The listing builds one solid part. Answer for the finished solid, in the listing's coordinates (mm). Face numbers are marked on the shaded views. A direction names the side the tool comes from. Round coordinates to 2 decimals unless told otherwise and drop trailing zeros. Loops run counter-clockwise (first coordinate to the right, second up) from the corner with the lowest first, then second, coordinate; pieces in that order, holes last. Notation, with made-up numbers: (40, -5) -> (78, -5) arc R27 cw to (78, 26) -> close; hole circle Ø1 at (-17.5, -15). An arc over 180 degrees is marked (long way). Use a Markdown table: item, result. Add a question column.
Q1. Section B-B on z = 25 is taken. Give the vertices of the cut face in (x, y).
Q2. Section A-A on x = 29.5 is taken. Give the vertices of the cut face in (y, z), then the cut area to 3 significant figures.
Q3. Consider line 1 (X direction, y = 5, z = 33); line 2 (Y direction, x = -16, z = 7.5); line 3 (X direction, y = 17, z = 5.5). Determine where each line is inside the solid, lowest interval first.
Q4. Section D-D on z = 5.5 is taken. Give the vertices of the cut face in (x, y).
Q5. For a pull along Y with two mould halves and no side action, classify the marked faces 3, 4 and 5 as released by +Y, released by -Y, zero draft, split by the parting line, or undercut.
Q6. Section C-C on y = 22 is taken. Give the vertices of the cut face in (x, z).
Q7. Given pin 1 Ø3 at (x, y) = (33, 14) entering from +Z; pin 2 Ø4 at (x, z) = (-42, 11.5) entering from +Y; pin 3 Ø1.8 at (x, z) = (-42.5, 9.5) entering from -Y, each flat-ended and moving along its own axis, determine where each tip first touches the part or whether it passes through.
Q8. Which of the six approach directions +Z, -Z, +X, -X, +Y, -Y give full straight-line access (tool end or side, diameter ignored) to the marked faces 1 and 2?
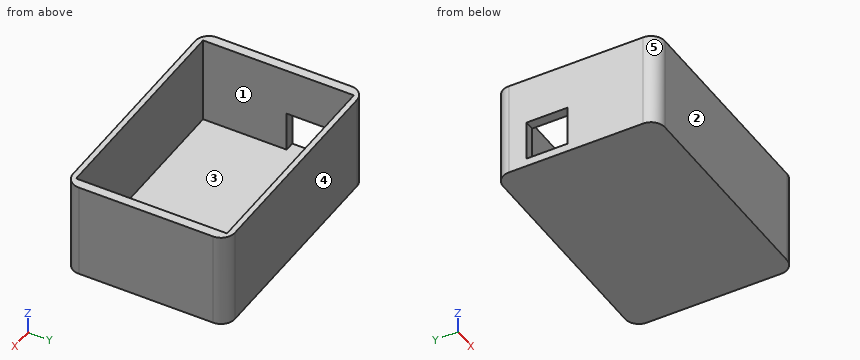
from build123d import *

# Parameters (mm, degrees)
F0_W     = 87
F0_H     = 59
F1_DEPTH = 35
F2_W     = 40
F2_H     = 27.5
F3_DEPTH = 32
F4_R     = 5
F5_W     = 15
F5_H     = 12.435101904
F5_H_2   = 2.1998170093
F6_DEPTH = 25


with BuildPart() as f1:
    # F0 (on Top) → F1 (new body)
    with BuildSketch(Plane.XY):
        Rectangle(F0_W, F0_H)
    extrude(amount=F1_DEPTH)

    # F2 (on face) → F3 (cut)
    with BuildSketch(Plane.XY.offset(35)):
        with Locations((-20, -13.75)):
            Rectangle(F2_W, F2_H)
        with Locations((20, 13.75)):
            Rectangle(F2_W, F2_H)
        with Locations((20, -13.75)):
            Rectangle(F2_W, F2_H)
        with Locations((-20, 13.75)):
            Rectangle(F2_W, F2_H)
    extrude(amount=-F3_DEPTH, mode=Mode.SUBTRACT)

    # F4
    f4_edges = [f1.edges().sort_by_distance(p)[0] for p in [
        (-43.5, -29.5, 17.5),
        (43.5, -29.5, 17.5),
        (43.5, 29.5, 17.5),
        (-43.5, 29.5, 17.5),
    ]]
    fillet(f4_edges, radius=F4_R)

    # F5 (on face) → F6 (cut)
    with BuildSketch(Plane(origin=(-43.5, 0, 0), x_dir=(0, -1, 0), z_dir=(-1, 0, 0))):
        with Locations((-10.5, 11.4173679613)):
            Rectangle(F5_W, F5_H)
        with Locations((-10.5, 4.0999085046)):
            Rectangle(F5_W, F5_H_2)
    extrude(amount=-F6_DEPTH, mode=Mode.SUBTRACT)


solid = f1.part
Checked values:
| question | item | result |
|---|---|---|
| 1 | outline | (-43.5, -24.5) arc R5 ccw to (-38.5, -29.5) -> (38.5, -29.5) arc R5 ccw to (43.5, -24.5) -> (43.5, 24.5) arc R5 ccw to (38.5, 29.5) -> (-38.5, 29.5) arc R5 ccw to (-43.5, 24.5) -> close; hole (-40, -27.5) -> (40, -27.5) -> (40, 27.5) -> (-40, 27.5) -> close |
| 2 | outline | (-29.5, 0) -> (29.5, 0) -> (29.5, 35) -> (27.5, 35) -> (27.5, 3) -> (-27.5, 3) -> (-27.5, 35) -> (-29.5, 35) -> close |
| 2 | area | 305 mm2 |
| 3 | line 1 | x = -43.5 to -40, 40 to 43.5 |
| 3 | line 2 | y = -29.5 to -27.5, 27.5 to 29.5 |
| 3 | line 3 | x = 40 to 43.5 |
| 4 | outline | (-43.5, -24.5) arc R5 ccw to (-38.5, -29.5) -> (38.5, -29.5) arc R5 ccw to (43.5, -24.5) -> (43.5, 24.5) arc R5 ccw to (38.5, 29.5) -> (-38.5, 29.5) arc R5 ccw to (-43.5, 24.5) -> (-43.5, 18) -> (-40, 18) -> (-40, 27.5) -> (40, 27.5) -> (40, -27.5) -> (-40, -27.5) -> (-40, 3) -> (-43.5, 3) -> close |
| 5 | face 3 | undercut |
| 5 | face 4 | released by +Y |
| 5 | face 5 | released by -Y |
| 6 | outline | (-43.5, 0) -> (43.5, 0) -> (43.5, 35) -> (40, 35) -> (40, 3) -> (-40, 3) -> (-40, 35) -> (-43.5, 35) -> close |
| 7 | pin 1 | stops at z = 3 |
| 7 | pin 2 | stops at y = 29.27 |
| 7 | pin 3 | stops at y = -28.42 |
| 8 | face 1 | +Z |
| 8 | face 2 | +Z, -Z, +X, -X, -Y |
